Check sheet for the modelled part. Datum: model origin and axes. Units: mm. Round coordinates to 2 decimals unless told otherwise and drop trailing zeros. Order: outer loops, then holes, each group sorted by start corner. A loop starts at its lowest first (then second) coordinate and runs counter-clockwise, first axis right, second up. Notation, with made-up numbers: (-18.5, 63.25) -> (-0.5, 63.25) arc R19 ccw to (-0.5, 72.25) -> close; hole circle Ø3 at (-34, 81). An arc over 180 degrees is marked (long way). Answer in a Markdown table with one row per item. Add a question column.
1. Material ranges on L1, parallel to Y at x = -52.5, z = 1.3; L2, parallel to Y at x = 8.5, z = 0.25; L3, parallel to X at y = -8.5, z = 1.2, recorded low to high. Write a range as from..to.
2. Depth check by flat-ended pin: P1, Ø9.5, axis at x = -7.5, y = 0, coming from the -Z side. Enter the tip coordinate at first touch or a pass-through.
3. Sectioned sample at D-D, the plane x = -51. Record the boundary of the cut face in (y, z), then the cut area to 3 significant figures.
4. Sectioned sample at B-B, the plane x = 37.5. Record the boundary of the cut face in (y, z), then the cut area to 3 significant figures.
5. Sectioned sample at A-A, the plane z = 1.65. Count the separate pieces of the cut face and the enclosed holes in it, then the cut area to 3 significant figures.
```python
from build123d import *

# Parameters (mm, degrees)
SKETCH3_R           = 3
BOSS_EXTRUDE1_DEPTH = 3


with BuildPart() as part:
    # Sketch3 → Boss-Extrude1 (new body)
    with BuildSketch(Plane.XY):
        with BuildLine():
            Line((-52.5, 10), (52.5, 10))
            ThreePointArc((52.5, 10), (62.5, 0), (52.5, -10))
            Line((52.5, -10), (-52.5, -10))
            ThreePointArc((-52.5, -10), (-62.5, 0), (-52.5, 10))
        make_face()
        with Locations((52.5, 0)):
            Circle(SKETCH3_R, mode=Mode.SUBTRACT)
        with Locations((-52.5, 0)):
            Circle(SKETCH3_R, mode=Mode.SUBTRACT)
        with Locations((-37.5, 0)):
            Circle(SKETCH3_R, mode=Mode.SUBTRACT)
        with Locations((-22.5, 0)):
            Circle(SKETCH3_R, mode=Mode.SUBTRACT)
        with Locations((-7.5, 0)):
            Circle(SKETCH3_R, mode=Mode.SUBTRACT)
        with Locations(Location((7.5, 0, 0), (0, 0, 180))):
            Circle(SKETCH3_R, mode=Mode.SUBTRACT)
        with Locations(Location((22.5, 0, 0), (0, 0, 180))):
            Circle(SKETCH3_R, mode=Mode.SUBTRACT)
        with Locations(Location((37.5, 0, 0), (0, 0, 180))):
            Circle(SKETCH3_R, mode=Mode.SUBTRACT)
    extrude(amount=BOSS_EXTRUDE1_DEPTH)


solid = part.part
```
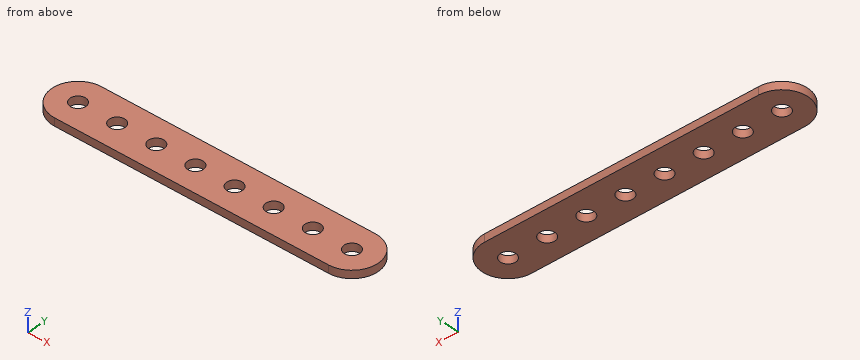
Answer key:
| question | item | result |
|---|---|---|
| 1 | L1 | y = -10..-3, 3..10 |
| 1 | L2 | y = -10..-2.83, 2.83..10 |
| 1 | L3 | x = -57.77..57.77 |
| 2 | P1 | stops at z = 0 |
| 3 | outline | (-10, 0) -> (-2.6, 0) -> (-2.6, 3) -> (-10, 3) -> close; (2.6, 0) -> (10, 0) -> (10, 3) -> (2.6, 3) -> close |
| 3 | area | 44.4 mm² |
| 4 | outline | (-10, 0) -> (-3, 0) -> (-3, 3) -> (-10, 3) -> close; (3, 0) -> (10, 0) -> (10, 3) -> (3, 3) -> close |
| 4 | area | 42.0 mm² |
| 5 | separate pieces | 1 |
| 5 | enclosed holes | 8 |
| 5 | area | 2,190 mm² |
